from build123d import *

# Parameters (mm, degrees)
SKETCH_2_W                       = 17
SKETCH_2_H                       = 15
SM_BASE_FLANGE_1_DEPTH           = 1.5
SM_EDGE_FLANGE_1_STRIP_W         = 7
SM_EDGE_FLANGE_1_STRIP_H         = 1.5
SM_EDGE_FLANGE_1_STRIP_CUT_DEPTH = 15
SM_EDGE_FLANGE_1_DEPTH           = 15
CUT_EXTRUDE_4_DEPTH              = 2
CUT_EXTRUDE_START                = -1.5
CUT_EXTRUDE_5_DEPTH              = 18.5


# Read off the part's stored shape, not the designer's step: 切除-拉伸5
# Sheet-metal steps are written as plain solids
with BuildPart() as part:
    # 草图2 → 基体-法兰1 (new body)
    with BuildSketch(Plane.XY):
        Rectangle(SKETCH_2_W, SKETCH_2_H)
    extrude(amount=SM_BASE_FLANGE_1_DEPTH)

    # 边线-法兰1 strip (across the edge) → 边线-法兰1 strip cut (cut)
    with BuildSketch(Plane(origin=(8.5, -7.5, 1.5), x_dir=(-1, 0, 0), z_dir=(0, 1, 0))):
        with Locations((-3, -0.75)):
            Rectangle(SM_EDGE_FLANGE_1_STRIP_W, SM_EDGE_FLANGE_1_STRIP_H)
    extrude(amount=SM_EDGE_FLANGE_1_STRIP_CUT_DEPTH, mode=Mode.SUBTRACT)

    # 边线-法兰1 section (across the edge) → 边线-法兰1 (add)
    with BuildSketch(Plane(origin=(8.5, -7.5, 1.5), x_dir=(-1, 0, 0), z_dir=(0, 1, 0))):
        with BuildLine():
            Line((-1.5, 0.5), (-1.5, 34))
            Line((-1.5, 34), (0, 34))
            Line((0, 34), (0, 0.5))
            ThreePointArc((0, 0.5), (0.146446609, 0.146446609), (0.5, 0))
            Line((0.5, 0), (0.5, -1.5))
            ThreePointArc((0.5, -1.5), (-0.914213562, -0.914213562), (-1.5, 0.5))
        make_face()
    extrude(amount=SM_EDGE_FLANGE_1_DEPTH)

    # 草图17 → 切除-拉伸4 (cut)
    with BuildSketch(Plane(origin=(8.5, 0, 0.26211679), x_dir=(0, 0, 1), z_dir=(-1, 0, 0))):
        Polygon((27.73788321, 6.01040764), (21.72747557, 0), (27.73788321, -6.01040764), (33.74829085, 0), align=None)
    extrude(amount=-CUT_EXTRUDE_4_DEPTH, mode=Mode.SUBTRACT)

    # 切除-拉伸5 outline → 切除-拉伸5 (cut)
    with BuildSketch(Plane(origin=(8.5, 0, 0.26211679), x_dir=(0, 0, 1), z_dir=(-1, 0, 0)).offset(CUT_EXTRUDE_START)):
        Polygon((1.73788321, 3.5), (24.454001029, 7.5), (-0.26211679, 7.5), (-0.26211679, 3.5), align=None)
        with BuildLine():
            Line((35.23788321, 7.5), (30.021765392, 7.5))
            ThreePointArc((30.021765392, 7.5), (33.805647573, 4.567764363), (35.23788321, 0))
            Line((35.23788321, 0), (35.23788321, 7.5))
        make_face()
        with BuildLine():
            Line((35.23788321, -7.5), (35.23788321, 0))
            ThreePointArc((35.23788321, 0), (33.805647573, -4.567764363), (30.021765392, -7.5))
            Line((30.021765392, -7.5), (35.23788321, -7.5))
        make_face()
        Polygon((-0.26211679, -7.5), (24.454001029, -7.5), (1.73788321, -3.5), (-0.26211679, -3.5), align=None)
    extrude(amount=CUT_EXTRUDE_5_DEPTH, mode=Mode.SUBTRACT)


solid = part.part
Check sheet for the modelled part. Datum: model origin and axes. Units: mm. A direction names the side the tool comes from. Round coordinates to 2 decimals unless told otherwise and drop trailing zeros. Loops run counter-clockwise (first coordinate to the right, second up) from the corner with the lowest first, then second, coordinate; pieces in that order, holes last. Notation, with made-up numbers: (46, 1) - (76, 1) arc R23 cw to (76, 21) - close; hole circle Ø8 at (35.25, 70). An arc over 180 degrees is marked (long way). Answer as CSV lines item,"result". Start each with the question number.
Item 1: Section check B-B (z = 26.5). Record the boundary of the cut face in (x, y).
Item 2: Release check for a two-part mould opening along Z. For faces 1 (the flat face through (9, -7.5, 28)), 2 (the flat face through (9.24, 3.05, 25.04)), 3 (the flat face through (0, 0, 0)) record: +Z half, -Z half, draft (parallel to the pull), parting line (faces both ways), or undercut.
Item 3: Section check C-C (y = 1.25). Record the boundary of the cut face in (x, z).
Item 4: Set-up check for faces 4 (the flat face through (0, 0, 1.5)), 5 (the flat face through (9.24, 2.96, 31.05)), 6 (the flat face through (1, -3.5, 1)): record each of +Z, -Z, +X, -X, +Y, -Y from which the full face is reachable in a straight line by a thin tool's end or side.
Item 5: Scan lines: line 1 (X direction, y = -6.5, z = 22); line 2 (Z direction, x = -2.75, y = 2.5); line 3 (Z direction, x = 9.25, y = 1.25). Record each from-to range of solid material in increasing order. Write a range as [from, to].
Item 6: Section check D-D (x = 3.25). Record the boundary of the cut face in (y, z), and give its area (3 significant figures).
Item 7: Section check A-A (y = -1.5). Record the boundary of the cut face in (x, z), and give its area (3 significant figures).
Item 8: Depth check by flat-ended pin: P1, Ø8, axis at y = -4.5, z = 14, coming from the -X side; P2, Ø2, axis at x = 0, z = 1, coming from the -Y side; P3, Ø2, axis at x = -4.5, y = 0.5, coming from the +Z side; P4, Ø3, axis at x = 6.5, z = 6, coming from the -Y side. Enter the tip coordinate at first touch or a pass-through.
Report:
1,outline,"(8.5, -7.5) - (10, -7.5) - (10, -4.51) - (8.5, -4.51) - close; (8.5, 4.51) - (10, 4.51) - (10, 7.5) - (8.5, 7.5) - close"
2,face 1,"draft"
2,face 2,"undercut"
2,face 3,"-Z half"
3,outline,"(-8.5, 0) - (8, 0) arc R2 ccw to (10, 2) - (10, 23.24) - (8.5, 23.24) - (8.5, 2) arc R0.5 cw to (8, 1.5) - (-8.5, 1.5) - close; (8.5, 32.76) - (10, 32.76) - (10, 35.4) - (8.5, 35.4) - close"
4,face 4,"+Z, -X, +Y, -Y"
4,face 5,"+X, -X"
4,face 6,"-Z, +X, -X, -Y"
5,line 1,"x = [8.5, 10]"
5,line 2,"z = [0, 1.5]"
5,line 3,"z = [0.44, 23.24], [32.76, 35.4]"
6,outline,"(-3.5, 0) - (3.5, 0) - (3.5, 1.5) - (-3.5, 1.5) - close"
6,area,"10.5 mm2"
7,outline,"(-8.5, 0) - (8, 0) arc R2 ccw to (10, 2) - (10, 23.49) - (8.5, 23.49) - (8.5, 2) arc R0.5 cw to (8, 1.5) - (-8.5, 1.5) - close; (8.5, 32.51) - (10, 32.51) - (10, 35.36) - (8.5, 35.36) - close"
7,area,"64.2 mm2"
8,P1,"stops at x = 8.5"
8,P2,"stops at y = -3.5"
8,P3,"stops at z = 1.5"
8,P4,"passes through"
